```python
from build123d import *
from build123d import SkipClean  # not in build123d's __all__

# Parameters (mm, degrees)
F0_R     = 5
F0_R_2   = 6
F0_R_3   = 9
F1_DEPTH = 28
F2_R     = 5
F2_R_2   = 6
F3_DEPTH = 10
F4_DEPTH = 25


with BuildPart() as f1:
    # F0 (on Top) → F1 (new body)
    with BuildSketch(Plane.XY):
        with BuildLine():
            ThreePointArc((14.102419126, 5.1109465654), (14.7739007525, 2.5945821542), (15, 0))
            ThreePointArc((15, 0), (10.6066017178, -10.6066017178), (0, -15))
            Line((0, -15), (0, -15.0284832917))
            Line((0, -15.0284832917), (-0.9230769231, -14.9715706923))
            ThreePointArc((-0.9230769231, -14.9715706923), (-15, 3.22e-08), (-0.9230768589, 14.9715706962))
            Line((-0.9230768589, 14.9715706962), (-65.6769230769, 10.979151841))
            ThreePointArc((-65.6769230769, 10.979151841), (-76, 0), (-65.6769230769, -10.979151841))
            Line((-65.6769230769, -10.979151841), (-11.6160346835, -14.3122930019))
            ThreePointArc((-11.6160346835, -14.3122930019), (-7.7343733546, -15.3615666346), (-4.5798065483, -17.8549535065))
            Line((-4.5798065483, -17.8549535065), (13.8787097995, -39.7917254502))
            ThreePointArc((13.8787097995, -39.7917254502), (24, -41.5692193817), (27.5212902005, -31.9151779832))
            Line((27.5212902005, -31.9151779832), (14.102419126, 5.1109465654))
        make_face()
        with Locations((20, -34.6410161514)):
            Circle(F0_R, mode=Mode.SUBTRACT)
        with Locations((-65, 0)):
            Circle(F0_R_2, mode=Mode.SUBTRACT)
        with BuildLine():
            ThreePointArc((0, -15), (10.6066017178, -10.6066017178), (15, 0))
            ThreePointArc((15, 0), (14.7739007525, 2.5945821542), (14.102419126, 5.1109465654))
            ThreePointArc((14.102419126, 5.1109465654), (8.2299296905, 12.5406641486), (-0.9230768589, 14.9715706962))
            ThreePointArc((-0.9230768589, 14.9715706962), (-15, 3.22e-08), (-0.9230769231, -14.9715706923))
            ThreePointArc((-0.9230769231, -14.9715706923), (-0.4617573041, -14.9928909885), (0, -15))
        make_face()
        Circle(F0_R_3, mode=Mode.SUBTRACT)
    extrude(amount=F1_DEPTH)

    # F2 (on face) → F3 (join)
    with BuildSketch(Plane.XY.offset(28)):
        with BuildLine():
            ThreePointArc((14.102419126, 5.1109465654), (14.7739007525, 2.5945821542), (15, 0))
            ThreePointArc((15, 0), (10.6066017178, -10.6066017178), (0, -15))
            Line((0, -15), (0, -15.0284832917))
            Line((0, -15.0284832917), (-0.9230769231, -14.9715706923))
            ThreePointArc((-0.9230769231, -14.9715706923), (-15, 3.22e-08), (-0.9230768589, 14.9715706962))
            Line((-0.9230768589, 14.9715706962), (-65.6769230769, 10.979151841))
            ThreePointArc((-65.6769230769, 10.979151841), (-76, 0), (-65.6769230769, -10.979151841))
            Line((-65.6769230769, -10.979151841), (-11.6160346835, -14.3122930019))
            ThreePointArc((-11.6160346835, -14.3122930019), (-7.7343733546, -15.3615666346), (-4.5798065483, -17.8549535065))
            Line((-4.5798065483, -17.8549535065), (13.8787097995, -39.7917254502))
            ThreePointArc((13.8787097995, -39.7917254502), (24, -41.5692193817), (27.5212902005, -31.9151779832))
            Line((27.5212902005, -31.9151779832), (14.102419126, 5.1109465654))
        make_face()
        with Locations((20, -34.6410161514)):
            Circle(F2_R, mode=Mode.SUBTRACT)
        with Locations((-65, 0)):
            Circle(F2_R_2, mode=Mode.SUBTRACT)
    extrude(amount=F3_DEPTH)

    # F4 (cut): a face of the model
    f4_faces = [f1.faces().sort_by_distance(p)[0] for p in [
        (-23.7772133401, -6.7537112781, 38),
    ]]
    with SkipClean():  # cleaning this boolean's faces spoils the solid; the shape is the same uncleaned
        extrude(f4_faces, amount=-F4_DEPTH, mode=Mode.SUBTRACT)


solid = f1.part
```
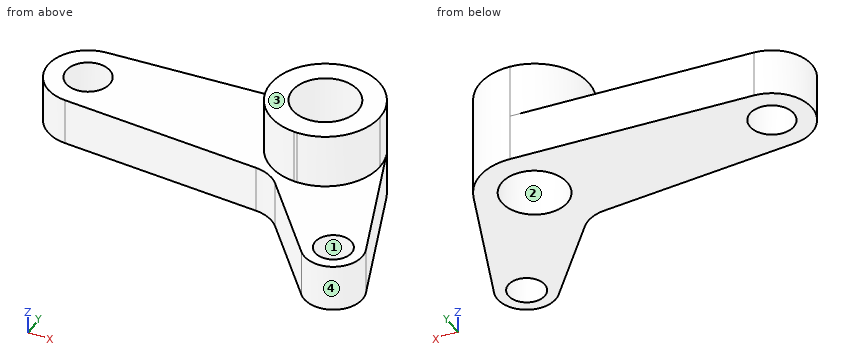
Geometry check sheet. Reference: the model listing, model coordinates, mm. Face numbers are marked on the shaded views. Give positions to 0.01 mm unless a question says otherwise; leave off trailing zeros. Order: outer loops, then holes, each group sorted by start corner. A loop starts at its lowest first (then second) coordinate and runs counter-clockwise, first axis right, second up. Notation, with made-up numbers: (-32, -34) - (21, -34) arc R13 ccw to (21, -27) - close; hole circle Ø9 at (-28.75, -16.5). An arc over 180 degrees is marked (long way). Write item = value, one per line. Start each with the question number.
1) Scan lines: L1, parallel to X at y = 3, z = 12; L2, parallel to Z at x = 17.5, y = -29.5; L3, parallel to Y at x = -65, z = 6.25. Record each from-to range of solid material in increasing order.
2) Section check C-C (y = -33). Enter the section's corners in (x, z).
3) Draft check along X on the marked faces 1, 2, 3 and 4. Enter one of: released by +X, released by -X, zero draft, split by the parting line, or undercut.
4) Gauge pin test, flat ends, axial feed: pin 1 Ø4 at (y, z) = (-17.5, 8) entering from -X; pin 2 Ø4 at (x, z) = (-6.5, 14) entering from -Y; pin 3 Ø8 at (y, z) = (3, 19.5) entering from -X. Record the tip position at first contact, or that the pin passes through.
5) Section check A-A (z = 21.75). Enter the section's corners in (x, y), then the cut area to 3 significant figures.
6) Section check D-D (x = 20). Enter the section's corners in (y, z), then the cut area to 3 significant figures.
7) Section check B-B (x = -3). Enter the section's corners in (y, z), then the cut area to 3 significant figures.
Geometry check:
q1.L1 = -75.58 to -70.2, -59.8 to -8.49, 8.49 to 14.87
q1.L2 = 0 to 13
q1.L3 = -11.02 to -6, 6 to 11.02
q2.outline = (8.16, 0) - (15.28, 0) - (15.28, 13) - (8.16, 13) - close; (24.72, 0) - (27.83, 0) - (27.83, 13) - (24.72, 13) - close
q3.face_1 = undercut
q3.face_2 = undercut
q3.face_3 = zero draft
q3.face_4 = split by the parting line
q4.pin_1 = -7.47
q4.pin_2 = -17.64
q4.pin_3 = -15
q5.outline = circle Ø30 at (0, 0); hole circle Ø18 at (0, 0)
q5.area = 452 mm2
q6.outline = (-42.64, 0) - (-39.64, 0) - (-39.64, 13) - (-42.64, 13) - close; (-29.64, 0) - (-11.16, 0) - (-11.16, 13) - (-29.64, 13) - close
q6.area = 279 mm2
q7.outline = (-19.73, 0) - (-8.49, 0) - (-8.49, 28) - (-14.7, 28) - (-14.7, 13) - (-19.73, 13) - close; (8.49, 0) - (14.84, 0) - (14.84, 13) - (14.7, 13) - (14.7, 28) - (8.49, 28) - close
q7.area = 415 mm2
